```python
from build123d import *

# Parameters (mm, degrees)
F1_DEPTH = 6.35
F2_D     = 4.826
F3_D     = 3.81
F4_SIZE2 = 6.3416783923
F4_SIZE  = 5.3213
F6_DEPTH = 25.4


# Not quite as in the source:
# - a feature names something its author has since deleted; it is built from what else it names


with BuildPart() as f1:
    # F0 (on Right) → F1 (new body)
    with BuildSketch(Plane.YZ):
        Polygon((274.6375, -12.7), (274.6375, 0), (274.6375, 53.8988), (0, 53.8988), (0, 0), (0, -12.7), align=None)
    extrude(amount=F1_DEPTH)

    # F2 (through all)
    with Locations(Plane(origin=(0, 0, 0), x_dir=(0, 1, 0), z_dir=(-1, 0, 0))):
        with Locations((4.7625, -40.4241), (4.7625, -26.9494), (4.7625, -13.4747)):
            Hole(F2_D / 2)

    # F3 (through all)
    with Locations(Plane(origin=(0, 0, 0), x_dir=(0, 1, 0), z_dir=(-1, 0, 0))):
        with Locations((271.4625, -40.4241), (271.4625, -26.9494), (271.4625, -13.4747)):
            Hole(F3_D / 2)

    # F4
    f4_edges = [f1.edges().sort_by_distance(p)[0] for p in [
        (6.35, 137.31875, 53.8988),
    ]]
    f4_side = f1.faces().sort_by_distance((6.35, 137.466328, 20.568323))[0]
    chamfer(f4_edges, length=F4_SIZE, length2=F4_SIZE2, reference=f4_side)

    # F5 (on face) → F6 (cut)
    with BuildSketch(Plane(origin=(0, 0, 0), x_dir=(0, -1, 0), z_dir=(-1, 0, 0))):
        Polygon((-274.6375, 53.8988), (-274.6375, 49.6316), (-249.2375, 49.6316), (-233.3625, 33.7566), (-41.275, 33.7566), (-25.4, 49.6316), (0, 49.6316), (0, 53.8988), align=None)
    extrude(amount=-F6_DEPTH, mode=Mode.SUBTRACT)


solid = f1.part
```
Could you check a few things on this model? Use its own coordinates, in mm. A direction names the side the tool comes from. Coordinates: 2 decimals unless noted, no trailing zeros. Loops run counter-clockwise (first coordinate to the right, second up) from the corner with the lowest first, then second, coordinate; pieces in that order, holes last.
1) Please list where these lines run through material, in increasing order: line 1 along Y through (x, z) = (4, 12); line 2 along Z through (x, y) = (1.75, 165); line 3 along Y through (x, z) = (5.5, 44.5).
Reported:
line 1: y = 0 to 2.85, 6.67 to 270.26, 272.67 to 274.64
line 2: z = -12.7 to 33.76
line 3: y = 0 to 30.53, 244.11 to 274.64
2) Which directions (+Z, -Z, +X, -X, +Y, -Y) give clear straight access to the entire face, cutting with the end or side of a thin tool? Please do faces 1 (the face through (3.13, 33.45, 41.58)), 2 (the face through (3, 135, -12.7)).
Reported:
face 1: +Z, +X, -X
face 2: -Z, +X, -X, +Y, -Y
3) Imagine slicing it at A-A (x = 3). List the corners of the cut face in (y, z) for me (1 decimal), and give its area (3 significant figures).
Reported:
outline: (0, -12.7) - (274.6, -12.7) - (274.6, 49.6) - (249.2, 49.6) - (233.4, 33.8) - (41.3, 33.8) - (25.4, 49.6) - (0, 49.6) - close; hole circle Ø4.8 at (4.8, 13.5); hole circle Ø4.8 at (4.8, 26.9); hole circle Ø4.8 at (4.8, 40.4); hole circle Ø3.8 at (271.5, 13.5); hole circle Ø3.8 at (271.5, 26.9); hole circle Ø3.8 at (271.5, 40.4)
area: 13,700 mm2
4) Imagine slicing it at B-B (y = 80). List the corners of the cut face in (x, z) for me.
Reported:
outline: (0, -12.7) - (6.35, -12.7) - (6.35, 33.76) - (0, 33.76) - close
5) Imagine slicing it at C-C (y = 243). List the corners of the cut face in (x, z) for me, and give its area (3 significant figures).
Reported:
outline: (0, -12.7) - (6.35, -12.7) - (6.35, 43.39) - (0, 43.39) - close
area: 356 mm2
6) Will these pins go through, and if not, where does the flat tip stop? pin 1 Ø3 at (x, y) = (4, 176) entering from +Z; pin 2 Ø2.5 at (y, z) = (271.46, 13.47) entering from -X.
Reported:
pin 1: stops at z = 33.76
pin 2: passes through
7) Thinking about a two-plate mould opening in Y: for faces 3 (the face through (6.35, 135, 12)), 4 (the face through (3, 0, 19)), 5 (the face through (3.22, 3.65, 29.09)), which applies, released by +Y, released by -Y, zero draft, split by the parting line, or undercut?
Reported:
face 3: zero draft
face 4: released by -Y
face 5: undercut
